```python
from build123d import *

# Parameters (mm, degrees)
EXTRUDE_1_DEPTH          = 5
SKETCH_2_R               = 2.1
SKETCH_2_R_2             = 2.6
CUT_EXTRUDE_1_DEPTH      = 10
PATTERN_CIRCULAR_1_COUNT = 3
EXTRUDE_3_DEPTH          = 5
SKETCH_6_R               = 5
CUT_EXTRUDE_2_DEPTH      = 285.979522771
CUT_EXTRUDE_4_DEPTH      = 285.979522771
CUT_EXTRUDE_5_DEPTH      = 242.721592744
CUT_EXTRUDE_6_DEPTH      = 10
FILLET_1_R               = 10
FILLET_2_R               = 10


with BuildPart() as part:
    # 草图1 → 凸台-拉伸1 (new body)
    with BuildSketch(Plane(origin=(0, 0, 0), x_dir=(1, 0, 0), z_dir=(0, 1, 0))):
        with BuildLine():
            Line((-34.641016151, 150), (-147.224318643, -45))
            ThreePointArc((-147.224318643, -45), (-147.224318643, -85), (-112.583302492, -105))
            Line((-112.583302492, -105), (112.583302492, -105))
            ThreePointArc((112.583302492, -105), (147.224318643, -85), (147.224318643, -45))
            Line((147.224318643, -45), (34.641016151, 150))
            ThreePointArc((34.641016151, 150), (0, 170), (-34.641016151, 150))
        make_face()
    extrude(amount=EXTRUDE_1_DEPTH)

    # 草图2 → 切除-拉伸1 (cut)
    with BuildSketch(Plane(origin=(0, 5, 0), x_dir=(1, 0, 0), z_dir=(0, 1, 0))):
        with Locations(Location((-10.75, 30, 0), (0, 0, 270))):
            Circle(SKETCH_2_R)
        with Locations(Location((-10.75, 134, 0), (0, 0, 270))):
            Circle(SKETCH_2_R)
        with Locations(Location((10.75, 30, 0), (0, 0, 270))):
            Circle(SKETCH_2_R)
        with Locations(Location((10.75, 134, 0), (0, 0, 270))):
            Circle(SKETCH_2_R)
        with Locations(Location((-36.38, 42, 0), (0, 0, 270))):
            Circle(SKETCH_2_R_2)
        with Locations(Location((-36.38, 122, 0), (0, 0, 270))):
            Circle(SKETCH_2_R_2)
        with Locations(Location((36.38, 122, 0), (0, 0, 270))):
            Circle(SKETCH_2_R_2)
        with Locations(Location((36.38, 42, 0), (0, 0, 270))):
            Circle(SKETCH_2_R_2)
    cut_extrude_1 = extrude(amount=-CUT_EXTRUDE_1_DEPTH, mode=Mode.SUBTRACT)

    # 阵列(圆周)1: 切除-拉伸1 ×3 about axis
    pattern_circular_1_axis = Axis((0, 0, 0.213703285), (0, 1, 0))
    for i in range(1, PATTERN_CIRCULAR_1_COUNT):
        add(cut_extrude_1.rotate(pattern_circular_1_axis, i * 360 / PATTERN_CIRCULAR_1_COUNT), mode=Mode.SUBTRACT)

    # 草图5 → 凸台-拉伸3 (add)
    with BuildSketch(Plane.XZ):
        with BuildLine():
            Line((69.282032303, -170), (181.865334795, 25))
            ThreePointArc((181.865334795, 25), (181.865334795, 105), (112.583302492, 145))
            Line((112.583302492, 145), (-112.583302492, 145))
            ThreePointArc((-112.583302492, 145), (-181.865334795, 105), (-181.865334795, 25))
            Line((-181.865334795, 25), (-69.282032303, -170))
            ThreePointArc((-69.282032303, -170), (0, -210), (69.282032303, -170))
        make_face()
        with BuildLine():
            Line((-147.224318643, 45), (-34.641016151, -150))
            ThreePointArc((-34.641016151, -150), (0, -170), (34.641016151, -150))
            Line((34.641016151, -150), (147.224318643, 45))
            ThreePointArc((147.224318643, 45), (147.224318643, 85), (112.583302492, 105))
            Line((112.583302492, 105), (-112.583302492, 105))
            ThreePointArc((-112.583302492, 105), (-147.224318643, 85), (-147.224318643, 45))
        make_face(mode=Mode.SUBTRACT)
    extrude(amount=-EXTRUDE_3_DEPTH)

    # 草图6 → 切除-拉伸2 (cut, through all)
    with BuildSketch(Plane(origin=(0, 5, 0), x_dir=(1, 0, 0), z_dir=(0, 1, 0))):
        with Locations(Location((-87.5, 119.5, 0), (0, 0, 270))):
            Circle(SKETCH_6_R)
        with Locations(Location((-87.5, 19.5, 0), (0, 0, 270))):
            Circle(SKETCH_6_R)
        with Locations(Location((87.5, 19.5, 0), (0, 0, 90))):
            Circle(SKETCH_6_R)
        with Locations(Location((87.5, 119.5, 0), (0, 0, 90))):
            Circle(SKETCH_6_R)
        with Locations(Location((-50, -18, 0), (0, 0, 90))):
            Circle(SKETCH_6_R)
        with Locations(Location((50, -18, 0), (0, 0, 270))):
            Circle(SKETCH_6_R)
    extrude(amount=-CUT_EXTRUDE_2_DEPTH, mode=Mode.SUBTRACT)

    # 草图8 → 切除-拉伸4 (cut, through all)
    with BuildSketch(Plane(origin=(0, 5, 0), x_dir=(1, 0, 0), z_dir=(0, 1, 0))):
        with BuildLine():
            Line((-83.138438763, 146), (83.138438763, 146))
            Line((83.138438763, 146), (69.282032303, 170))
            ThreePointArc((69.282032303, 170), (0, 210), (-69.282032303, 170))
            Line((-69.282032303, 170), (-83.138438763, 146))
        make_face()
    extrude(amount=-CUT_EXTRUDE_4_DEPTH, mode=Mode.SUBTRACT)

    # 草图9 → 切除-拉伸5 (cut, through all)
    with BuildSketch(Plane(origin=(0, 5, 0), x_dir=(1, 0, 0), z_dir=(0, 1, 0))):
        with BuildLine():
            Line((-132.501886779, 60.5), (-132.501886779, -82.5))
            Line((-132.501886779, -82.5), (-67.549981495, -120))
            Line((-67.549981495, -120), (67.549981495, -120))
            Line((67.549981495, -120), (132.501886779, -82.5))
            Line((132.501886779, -82.5), (132.501886779, 60.5))
            Line((132.501886779, 60.5), (181.865334795, -25))
            ThreePointArc((181.865334795, -25), (181.865334795, -105), (112.583302492, -145))
            Line((112.583302492, -145), (-112.583302492, -145))
            ThreePointArc((-112.583302492, -145), (-181.865334795, -105), (-181.865334795, -25))
            Line((-181.865334795, -25), (-132.501886779, 60.5))
        make_face()
    extrude(amount=-CUT_EXTRUDE_5_DEPTH, mode=Mode.SUBTRACT)

    # 草图10 → 切除-拉伸6 (cut)
    with BuildSketch(Plane.XZ):
        with BuildLine():
            Line((-132.501886779, 11), (-132.501886779, -60.5))
            Line((-132.501886779, -60.5), (-107.820162771, -103.25))
            ThreePointArc((-107.820162771, -103.25), (-95.363092594, -40.767838354), (-132.501886779, 11))
        make_face()
        with BuildLine():
            Line((132.501886779, 11), (132.501886779, -60.5))
            Line((132.501886779, -60.5), (107.820162771, -103.25))
            ThreePointArc((107.820162771, -103.25), (95.363092594, -40.767838354), (132.501886779, 11))
        make_face()
        Polygon((0, -93.759719881), (0, -117.74775549), (15.192422552, -125.743767359), (15.192422552, -101.755731751), align=None)
        Polygon((-11.727484075, -82.032235806), (-35.715519683, -82.032235806), (-43.711531553, -97.224658358), (-19.723495945, -97.224658358), align=None)
        Polygon((0, -70.304751731), (0, -46.316716123), (-15.192422552, -38.320704253), (-15.192422552, -62.308739862), align=None)
        Polygon((11.727484075, -82.032235806), (35.715519683, -82.032235806), (43.711531553, -66.839813254), (19.723495945, -66.839813254), align=None)
        with BuildLine():
            Line((-109.888608331, 15.515490775), (-70.976675957, 0.514623515))
            ThreePointArc((-70.976675957, 0.514623515), (-57.594007807, 41.483534468), (-22.975810906, 67.157021081))
            Line((-22.975810906, 67.157021081), (-35.715519683, 105.074441939))
            ThreePointArc((-35.715519683, 105.074441939), (-85.471293176, 70.78767363), (-109.888608331, 15.515490775))
        make_face()
        with BuildLine():
            Line((109.888608331, 15.515490775), (70.976675957, 0.514623515))
            ThreePointArc((70.976675957, 0.514623515), (57.594007807, 41.483534468), (22.975810906, 67.157021081))
            Line((22.975810906, 67.157021081), (35.715519683, 105.074441939))
            ThreePointArc((35.715519683, 105.074441939), (85.471293176, 70.78767363), (109.888608331, 15.515490775))
        make_face()
    extrude(amount=-CUT_EXTRUDE_6_DEPTH, mode=Mode.SUBTRACT)

    # 圆角1
    fillet_1_edges = [part.edges().sort_by_distance(p)[0] for p in [
        (-83.138438763, 2.5, -146),
        (-132.501886779, 2.5, 82.5),
        (-132.501886779, 2.5, 11),
        (-107.820162771, 2.5, -103.25),
    ]]
    fillet(fillet_1_edges, radius=FILLET_1_R)

    # 圆角2
    fillet_2_edges = [part.edges().sort_by_distance(p)[0] for p in [
        (83.138438763, 2.5, -146),
        (-67.549981495, 2.5, 120),
        (67.549981495, 2.5, 120),
        (132.501886779, 2.5, 82.5),
        (132.501886779, 2.5, 11),
        (107.820162771, 2.5, -103.25),
    ]]
    fillet(fillet_2_edges, radius=FILLET_2_R)


solid = part.part
```
Could you check a few things on this model? Use its own coordinates, in mm. A direction names the side the tool comes from. Round coordinates to 2 decimals unless told otherwise and drop trailing zeros. Loops run counter-clockwise (first coordinate to the right, second up) from the corner with the lowest first, then second, coordinate; pieces in that order, holes last. Notation, with made-up numbers: (54.5, 5) - (76.5, 5) arc R23 ccw to (76.5, 20) - close; hole circle Ø10 at (-21.5, -0.75). An arc over 180 degrees is marked (long way). Answer in a Markdown table with one row per item. Add a question column.
(1) If we section it at A-A (z = 101): Please give me the cut outline in (x, y).
(2) If we mould it in two halves opening along X, with no side actions, what happens to faces 3 (the face through (-99.09, 2.54, 101.79)), 4 (the face through (98.28, 2.54, 102.26)), 5 (the face through (-7.7, 2.46, -66.25)), 6 (the face through (84.92, 2.46, 71.45))? For each: pulls with the +X half, pulls with the -X half, needs draft (parallel to the pull), parting line crosses it, or undercut.
(3) I'm going to push flat-ended pins straight in: pin 1 (8.5 mm diameter, centred on x = 54.75, z = -10.19, fed in from -Y); pin 2 (1 mm diameter, centred on y = 2, z = 90.5, fed in from +X); pin 3 (2 mm diameter, centred on x = -69, y = 3.5, fed in from +Z); pin 4 (2 mm diameter, centred on x = -101.5, y = 2, fed in from +Z). Where does each tip first touch, or does it pass through?
(4) For faces 1 (the face through (-29.256, 2.465, 85.85)), 2 (the face through (95.25, 2.46, -41.3)), which set-ups out of +Z, -Z, +X, -X, +Y, -Y let a thin tool reach every point of the face, with its end or its side?
(5) If we section it at B-B (y = 3.45): State how many separate pieces and enclosed holes the cut face has, plus the area to 3 significant figures.
(6) I need wall thicknesses on line 1 along X through (y, z) = (1.8, 20); line 2 along X through (y, z) = (0.5, -122); line 3 along X through (y, z) = (0.9, -55). Which ranges of each line are inside material? Lowest first, please.
Model answer:
| question | item | result |
|---|---|---|
| 1 | outline | (-100.46, 0) - (-45.99, 0) - (-45.99, 5) - (-100.46, 5) - close; (-34.35, 0) - (34.35, 0) - (34.35, 5) - (-34.35, 5) - close; (45.99, 0) - (100.46, 0) - (100.46, 5) - (45.99, 5) - close |
| 2 | face 3 | pulls with the -X half |
| 2 | face 4 | pulls with the +X half |
| 2 | face 5 | undercut |
| 2 | face 6 | undercut |
| 3 | pin 1 | stops at y = 0 |
| 3 | pin 2 | stops at x = 119.51 |
| 3 | pin 3 | stops at z = 119.5 |
| 3 | pin 4 | stops at z = 100.98 |
| 4 | face 1 | +Y, -Y |
| 4 | face 2 | +X, +Y, -Y |
| 5 | separate pieces | 1 |
| 5 | enclosed holes | 36 |
| 5 | area | 47,200 mm² |
| 6 | line 1 | x = -132.5 to -109.16, -68.1 to -54.58, -45.42 to 45.42, 54.58 to 68.1, 109.16 to 132.5 |
| 6 | line 2 | x = -96.99 to -91.83, -83.17 to -38.98, -33.78 to 8.08, 15.19 to 33.78, 38.98 to 83.17, 91.83 to 96.99 |
| 6 | line 3 | x = -93.6 to -15.19, 0 to 93.6 |
